Geometry: final body of the model. Coordinates: model frame, mm. Face numbers are marked on the shaded views. Give positions to 0.01 mm unless a question says otherwise; leave off trailing zeros. Write each loop counter-clockwise with the first axis right and the second up, starting at its lowest first coordinate (ties: lowest second). Pieces come first, ordered by that corner, then holes. Notation, with made-up numbers: (-22.5, 2.25) - (25.5, 2.25) arc R16 ccw to (25.5, 12.25) - close; hole circle Ø2 at (66.5, 40). An arc over 180 degrees is marked (long way). Use CSV: the item, a comma, the result in double quotes. Start each with the question number.
(1) First-contact query: pin 1 Ø1.5 at (x, y) = (14, 7.5) entering from +Z; pin 2 Ø1.5 at (y, z) = (6, 3.5) entering from +X. Flat tips, straight axial feed; report the tip coordinate or a pass-through.
(2) Draft query along Y for the marked faces 1, 2 and 3. Return one class per face: released by +Y, released by -Y, zero draft, split by the parting line, or undercut.
(3) Section C-C on z = 2. Output: boundary loops of the cut face in (x, y), and give its area (3 significant figures).
(4) Section D-D on z = 4. Output: boundary loops of the cut face in (x, y), and give its area (3 significant figures).
(5) Section B-B on y = 7.5. Output: boundary loops of the cut face in (x, z).
(6) Line query: probe 1 along Y at (x, z) = (14, 4.15); probe 2 along Z at (x, y) = (13.25, 8.2); probe 3 along X at (y, z) = (8.25, 1.15). Output: solid intervals per line, ascending. Write a range as [from, to].
(7) Section A-A on x = 14. Output: boundary loops of the cut face in (y, z), and give its area (3 significant figures).
from build123d import *

# Parameters (mm, degrees)
CYLINDER008_R     = 1.25
CYLINDER008_DEPTH = 5
CYLINDER019_R     = 3
CYLINDER019_DEPTH = 6


with BuildPart() as obj1:
    # Cylinder008 → Cylinder008 (new body)
    with BuildSketch(Plane(origin=(50, 14, 3), x_dir=(1, 0, 0), z_dir=(0, 0, 1))):
        Circle(CYLINDER008_R)
    extrude(amount=CYLINDER008_DEPTH)


with BuildPart() as h_cut009:
    # Cylinder019 → Cylinder019 (new body)
    with BuildSketch(Plane(origin=(50, 14, 0), x_dir=(1, 0, 0), z_dir=(0, 0, 1))):
        Circle(CYLINDER019_R)
    extrude(amount=CYLINDER019_DEPTH)

    # Cut009: cut obj1
    add(obj1.part, mode=Mode.SUBTRACT)


with BuildPart() as h_cut009_1:
    # Cut009 placement: moved
    add(h_cut009.part.moved(Location((-36, -6.5, 0))))


solid = h_cut009_1.part
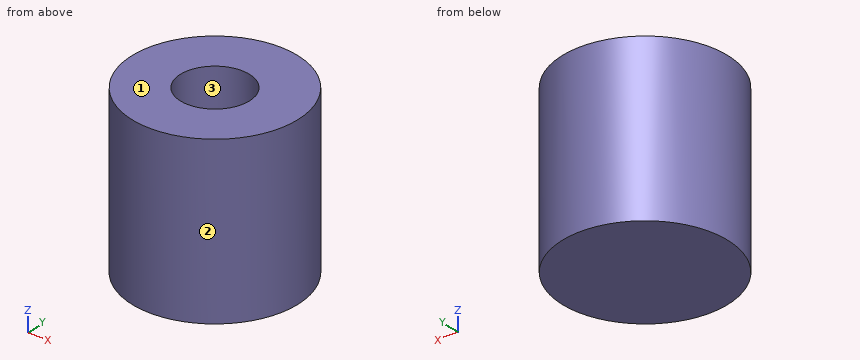
Check values:
1,pin 1,"stops at z = 3"
1,pin 2,"stops at x = 16.9"
2,face 1,"zero draft"
2,face 2,"split by the parting line"
2,face 3,"undercut"
3,outline,"circle Ø6 at (14, 7.5)"
3,area,"28.3 mm²"
4,outline,"circle Ø6 at (14, 7.5); hole circle Ø2.5 at (14, 7.5)"
4,area,"23.4 mm²"
5,outline,"(11, 0) - (17, 0) - (17, 6) - (15.25, 6) - (15.25, 3) - (12.75, 3) - (12.75, 6) - (11, 6) - close"
6,probe 1,"y = [4.5, 6.25], [8.75, 10.5]"
6,probe 2,"z = [0, 3]"
6,probe 3,"x = [11.1, 16.9]"
7,outline,"(4.5, 0) - (10.5, 0) - (10.5, 6) - (8.75, 6) - (8.75, 3) - (6.25, 3) - (6.25, 6) - (4.5, 6) - close"
7,area,"28.5 mm²"
